```python
from build123d import *

# Parameters (mm, degrees)
F0_R     = 21.59
F0_R_2   = 20.6375
F1_DEPTH = 12.7
F2_R     = 21.59
F3_DEPTH = 12.7
F3_TAPER = 45
F4_R     = 0.762
F5_R     = 6.35
F6_DEPTH = 25.4
F7_SIZE  = 0.762


with BuildPart() as f1:
    # F0 (on Front) → F1 (new body)
    with BuildSketch(Plane.XZ):
        Circle(F0_R)
        Circle(F0_R_2, mode=Mode.SUBTRACT)
    extrude(amount=F1_DEPTH)

    # F2 (on face) → F3 (join)
    with BuildSketch(Plane.XZ.offset(12.7)):
        Circle(F2_R)
    extrude(amount=F3_DEPTH, taper=F3_TAPER)

    # F4
    f4_edges = [f1.edges().sort_by_distance(p)[0] for p in [
        (-21.59, -12.7, 0),
        (-8.89, -25.4, 0),
    ]]
    fillet(f4_edges, radius=F4_R)

    # F5 (on face) → F6 (cut)
    with BuildSketch(Plane.XZ.offset(25.4)):
        Circle(F5_R)
    extrude(amount=-F6_DEPTH, mode=Mode.SUBTRACT)

    # F7
    f7_edges = [f1.edges().sort_by_distance(p)[0] for p in [
        (-6.35, -25.4, 0),
        (-20.6375, 0, 0),
    ]]
    chamfer(f7_edges, length=F7_SIZE)


solid = f1.part
```
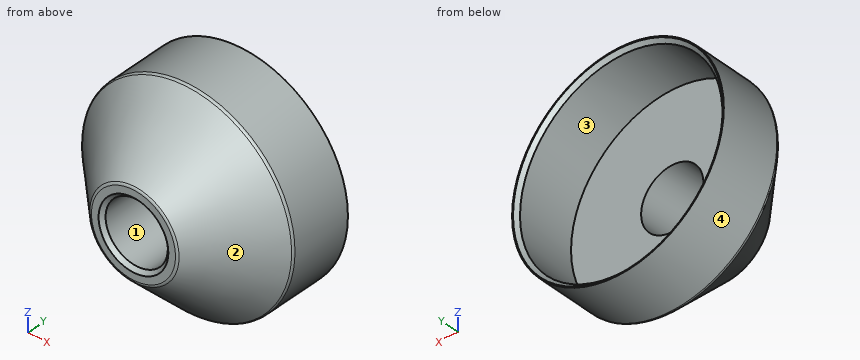
Verification items for the finished model (mm, model axes). Face numbers are marked on the shaded views. A direction names the side the tool comes from. Coordinates: 2 decimals unless noted, no trailing zeros. Loops run counter-clockwise (first coordinate to the right, second up) from the corner with the lowest first, then second, coordinate; pieces in that order, holes last. Notation, with made-up numbers: (59, 16.25) -> (92, 16.25) arc R11 cw to (92, 22.25) -> close; hole circle Ø8 at (49.25, -4.75). An arc over 180 degrees is marked (long way). Answer in a Markdown table with one row per item. Add a question column.
1. Material ranges on probe 1 along Y at (x, z) = (8, -1.5); probe 2 along Z at (x, y) = (0, -19.5); probe 3 along Z at (x, y) = (-15, -3.75), recorded low to high. Write a range as [from, to].
2. Access from +Z, -Z, +X, -X, +Y, -Y to the whole of each face (thin tool, end or side, straight path). Record for the marked faces 3 and 4.
3. Depth check by flat-ended pin: P1, Ø3, axis at x = 9.5, y = -14.5, coming from the +Z side; P2, Ø4, axis at x = 8.5, z = -8, coming from the -Y side; P3, Ø10, axis at y = -15, z = -5.5, coming from the -X side. Enter the tip coordinate at first touch or a pass-through.
4. Section check A-A, the plane y = -23.5. Enter the section's corners in (x, z).
5. Draft check along X on the marked faces 1 and 2. Enter one of: +X half, -X half, draft (parallel to the pull), parting line (faces both ways), or undercut.
6. Section check B-B, the plane y = -17. Enter the section's corners in (x, z), then the cut area to 3 significant figures.
Derived:
| question | item | result |
|---|---|---|
| 1 | probe 1 | y = [-25.4, -12.7] |
| 1 | probe 2 | z = [-14.79, -6.35], [6.35, 14.79] |
| 1 | probe 3 | z = [-15.53, -14.17], [14.17, 15.53] |
| 2 | face 3 | +Y |
| 2 | face 4 | +Y, -Y |
| 3 | P1 | stops at z = 19.2 |
| 3 | P2 | stops at y = -24.62 |
| 3 | P3 | stops at x = -21.55 |
| 4 | outline | circle Ø21.58 at (0, 0); hole circle Ø12.7 at (0, 0) |
| 5 | face 1 | undercut |
| 5 | face 2 | parting line |
| 6 | outline | circle Ø34.58 at (0, 0); hole circle Ø12.7 at (0, 0) |
| 6 | area | 812 mm² |
